```python
from build123d import *

# Parameters (mm, degrees)
F0_W     = 110
F0_H     = 20
F0_H_2   = 90
F1_DEPTH = 4
F2_DEPTH = 20
F4_DEPTH = 100
F3_R     = 8
F5_DEPTH = 77
F6_R     = 10
F6_R_2   = 8
F7_DEPTH = 2
F8_W     = 75
F8_H     = 5
F9_DEPTH = 25


# Not quite as in the source:
# - a pattern or mirror of a feature is missing from the dataset's text; its kind, count and spacing are read off the source's solid
# - a feature names something its author has since deleted; it is built from what else it names


with BuildPart() as f1:
    # F0 (on Top) → F1 (new body)
    with BuildSketch(Plane.XY):
        with Locations((0, -55)):
            Rectangle(F0_W, F0_H)
        Rectangle(F0_W, F0_H_2)
    extrude(amount=F1_DEPTH)

    # F0 (on Top) → F2 (join)
    with BuildSketch(Plane.XY):
        with Locations((0, -55)):
            Rectangle(F0_W, F0_H)
    extrude(amount=F2_DEPTH)

    # F3 (on Right) → F4 (cut, symmetric)
    with BuildSketch(Plane.YZ):
        with BuildLine():
            Line((-65, 2), (-65, 0))
            Line((-65, 0), (-55, 0))
            ThreePointArc((-55, 0), (-62.0710678119, 2.9289321881), (-65, 10))
            Line((-65, 10), (-65, 2))
        make_face()
        with BuildLine():
            Line((-65, 20), (-65, 10))
            ThreePointArc((-65, 10), (-62.0710678119, 17.0710678119), (-55, 20))
            Line((-55, 20), (-65, 20))
        make_face()
        with BuildLine():
            ThreePointArc((-55, 20), (-47.9289321881, 17.0710678119), (-45, 10))
            Line((-45, 10), (-45, 20))
            Line((-45, 20), (-55, 20))
        make_face()
    extrude(amount=F4_DEPTH, both=True, mode=Mode.SUBTRACT)

    # F3 (on Right) → F5 (join, symmetric)
    with BuildSketch(Plane.YZ):
        with Locations((-55, 10)):
            Circle(F3_R)
    extrude(amount=F5_DEPTH, both=True)

    # F6 (on face) → F7 (join)
    with BuildSketch(Plane(origin=(-77, 0, 0), x_dir=(0, -1, 0), z_dir=(-1, 0, 0))):
        with Locations((55, 10)):
            Circle(F6_R)
        with Locations((55, 10)):
            Circle(F6_R_2, mode=Mode.SUBTRACT)
        with Locations((55, 10)):
            Circle(F6_R_2)
    f7 = extrude(amount=F7_DEPTH)

    # F7_copies: F7 across plane
    add(f7.mirror(Plane(origin=(0, 0, 0), x_dir=(0, 0, 1), z_dir=(1, 0, 0))))

    # F8 (on face) → F9 (cut)
    with BuildSketch(Plane.XY.offset(4)):
        with Locations((0, 3.5)):
            Rectangle(F8_W, F8_H)
        with Locations((0, 10.5)):
            Rectangle(F8_W, F8_H)
        with Locations((0, 31.5)):
            Rectangle(F8_W, F8_H)
        with Locations((0, 24.5)):
            Rectangle(F8_W, F8_H)
        with Locations((0, 17.5)):
            Rectangle(F8_W, F8_H)
        with Locations((0, 38.5)):
            Rectangle(F8_W, F8_H)
        Polygon((37.5, -8), (37.5, -6), (37.5, -1), (-37.5, -1), (-37.5, -6), (-37.5, -8), (-37.5, -13), (-37.5, -15), (-37.5, -20), (-37.5, -22), (-37.5, -27), (-37.5, -29), (-37.5, -34), (-37.5, -36), (-37.5, -41), (37.5, -41), (37.5, -36), (37.5, -34), (37.5, -29), (37.5, -27), (37.5, -22), (37.5, -20), (37.5, -15), (37.5, -13), align=None)
    extrude(amount=-F9_DEPTH, mode=Mode.SUBTRACT)


solid = f1.part
```
Build history of the part. All positions in model axes, mm. A direction names the side the tool comes from. Give positions to 0.01 mm unless a question says otherwise; leave off trailing zeros. Loops run counter-clockwise (first coordinate to the right, second up) from the corner with the lowest first, then second, coordinate; pieces in that order, holes last.
1) Band-saw the part on B-B on x = 26. State how many separate pieces and enclosed holes the cut face has, then the cut area to 3 significant figures.
Values follow:
separate pieces: 8
enclosed holes: 0
area: 416 mm2
2) Probe line 1 along X through (y, z) = (-6, 3.25); line 2 along Y through (x, z) = (7.5, 9.25); line 3 along Z through (x, y) = (-32, 7). List the from-to ranges inside material, lowest first.
Values follow:
line 1: x = -55 to -37.5, 37.5 to 55
line 2: y = -64.97 to -45
line 3: z = 0 to 4
3) Band-saw the part on C-C on z = 16.25. List the corners of the cut face in (x, y), then the cut area to 3 significant figures.
Values follow:
outline: (-79, -62.81) - (-77, -62.81) - (-77, -59.99) - (-55, -59.99) - (-55, -62.81) - (55, -62.81) - (55, -59.99) - (77, -59.99) - (77, -62.81) - (79, -62.81) - (79, -47.19) - (77, -47.19) - (77, -50.01) - (55, -50.01) - (55, -47.19) - (-55, -47.19) - (-55, -50.01) - (-77, -50.01) - (-77, -47.19) - (-79, -47.19) - close
area: 2,220 mm2
4) Two-plate mould, pull along Y, no slides. Class faces 5 (the face through (-1, 15, 2)), 6 (the face through (-37.5, 24, 2)), 7 (the face through (78, -45, 10)), 8 (the face through (-1, -45, 7)): released by +Y, released by -Y, zero draft, split by the parting line, or undercut.
Values follow:
face 5: undercut
face 6: undercut
face 7: split by the parting line
face 8: released by +Y
5) Drop flat-ended pins along their axis: P1, Ø2, axis at x = 47.5, z = 2, coming from the -Y side; P2, Ø12, axis at x = 20, y = -5, coming from the +Z side; P3, Ø10, axis at x = -26.5, z = 2.5, coming from the -Y side; P4, Ø1, axis at x = 34.5, y = 11.5, coming from the -Z side. Give the stop position or say it passes through.
Values follow:
P1: stops at y = -62.14
P2: stops at z = 4
P3: stops at y = -64.68
P4: passes through
6) 3-axis set-ups, long thin cutter, end or side, ignore diameter. For faces 1 (the face through (77, -55, 18.2)), 2 (the face through (-1, 7, 0)), 3 (the face through (-78, -45, 10)), 4 (the face through (-37.5, 10, 2)): which of +Z, -Z, +X, -X, +Y, -Y reach the whole face in a straight line?
Values follow:
face 1: none
face 2: -Z, +X, -X, +Y, -Y
face 3: -X
face 4: +Z, -Z
7) Band-saw the part on A-A on y = -3.5. List the corners of the cut face in (x, z).
Values follow:
outline: (-55, 0) - (-37.5, 0) - (-37.5, 4) - (-55, 4) - close; (37.5, 0) - (55, 0) - (55, 4) - (37.5, 4) - close
